Work out the finished part from the listing and answer in its coordinate system (mm). Face numbers are marked on the shaded views. Round coordinates to 2 decimals unless told otherwise and drop trailing zeros. Loops run counter-clockwise (first coordinate to the right, second up) from the corner with the lowest first, then second, coordinate; pieces in that order, holes last. Notation, with made-up numbers: (81.25, 52.5) - (119.25, 52.5) arc R21 cw to (119.25, 57.5) - close; hole circle Ø10 at (-30, 52). An arc over 180 degrees is marked (long way). Answer as CSV lines item,"result". Start each with the question number.
Q1. Section C-C on y = 0 is taken. Write down the section's boundary in (x, z).
Q2. Each of these flat-tipped pins is pushed along its axis until it touches: pin 1 Ø10 at (y, z) = (10, 6.5) entering from -X; pin 2 Ø3 at (x, z) = (1, 11) entering from +Y; pin 3 Ø1.5 at (y, z) = (-9, 18.5) entering from +X; pin 4 Ø12 at (x, z) = (17.5, 16.5) entering from +Y. Where does it stop, or does it pass through?
Q3. Straight lines are drawn through the part: L1, parallel to Y at x = -20, z = 1.7 (3 decimals); L2, parallel to Y at x = 0.5, z = 18.5; L3, parallel to Z at x = -14, y = -19. For each, find the intervals that lie inside material, in ascending order. Write a range as [from, to].
Q4. Section A-A on y = 20 is taken. Write down the section's boundary in (x, z) (3 decimals), then the cut area to 3 significant figures.
Q5. The mould has two halves that part along Z. Classify the marked faces 1, 2 and 3: +Z half, -Z half, draft (parallel to the pull), parting line (faces both ways), or undercut.
```python
from build123d import *

# Parameters (mm, degrees)
F0_W     = 53
F0_H     = 53
F0_R     = 2.025
F0_R_2   = 12.5
F0_R_3   = 9.5
F1_DEPTH = 3
F2_DEPTH = 28
F3_R     = 2
F4_R     = 3
F5_R     = 2


with BuildPart() as f1:
    # F0 (on Top) → F1 (new body)
    with BuildSketch(Plane.XY):
        Rectangle(F0_W, F0_H)
        with Locations((-20, -20)):
            Circle(F0_R, mode=Mode.SUBTRACT)
        with Locations((20, -20)):
            Circle(F0_R, mode=Mode.SUBTRACT)
        with Locations((-20, 20)):
            Circle(F0_R, mode=Mode.SUBTRACT)
        Circle(F0_R_2, mode=Mode.SUBTRACT)
        with Locations((20, 20)):
            Circle(F0_R, mode=Mode.SUBTRACT)
        Circle(F0_R_2)
        Circle(F0_R_3, mode=Mode.SUBTRACT)
    extrude(amount=F1_DEPTH)

    # F0 (on Top) → F2 (join)
    with BuildSketch(Plane.XY):
        Circle(F0_R_2)
        Circle(F0_R_3, mode=Mode.SUBTRACT)
    extrude(amount=F2_DEPTH)

    # F3
    f3_edges = [f1.edges().sort_by_distance(p)[0] for p in [
        (-12.5, 0, 28),
    ]]
    fillet(f3_edges, radius=F3_R)

    # F4
    f4_edges = [f1.edges().sort_by_distance(p)[0] for p in [
        (-12.5, 0, 3),
    ]]
    fillet(f4_edges, radius=F4_R)

    # F5
    f5_edges = [f1.edges().sort_by_distance(p)[0] for p in [
        (-26.5, -26.5, 1.5),
        (26.5, -26.5, 1.5),
        (26.5, 26.5, 1.5),
        (-26.5, 26.5, 1.5),
    ]]
    fillet(f5_edges, radius=F5_R)


solid = f1.part
```
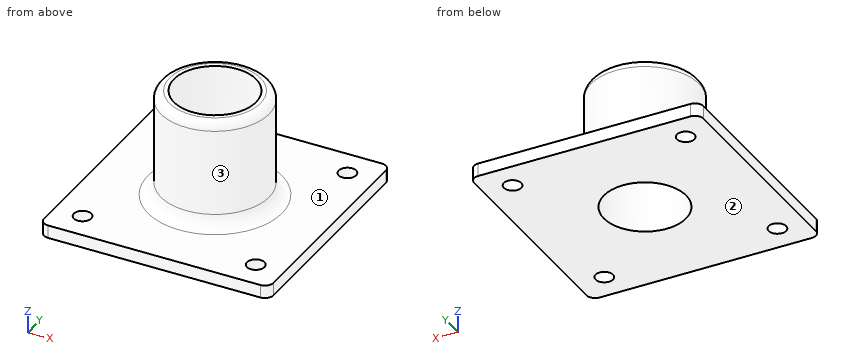
Findings:
1,outline,"(-26.5, 0) - (-9.5, 0) - (-9.5, 28) - (-10.5, 28) arc R2 ccw to (-12.5, 26) - (-12.5, 6) arc R3 cw to (-15.5, 3) - (-26.5, 3) - close; (9.5, 0) - (26.5, 0) - (26.5, 3) - (15.5, 3) arc R3 cw to (12.5, 6) - (12.5, 26) arc R2 ccw to (10.5, 28) - (9.5, 28) - close"
2,pin 1,"stops at x = -26.5"
2,pin 2,"stops at y = 12.5"
2,pin 3,"stops at x = 9.39"
2,pin 4,"stops at y = 4.9"
3,L1,"y = [-26.5, -22.025], [-17.975, 17.975], [22.025, 26.5]"
3,L2,"y = [-12.49, -9.49], [9.49, 12.49]"
3,L3,"z = [0, 3]"
4,outline,"(-26.5, 0) - (-22.025, 0) - (-22.025, 3) - (-26.5, 3) - close; (-17.975, 0) - (17.975, 0) - (17.975, 3) - (-17.975, 3) - close; (22.025, 0) - (26.5, 0) - (26.5, 3) - (22.025, 3) - close"
4,area,"135 mm^2"
5,face 1,"+Z half"
5,face 2,"-Z half"
5,face 3,"draft"
